from build123d import *

# Parameters (mm, degrees)
ESBO_O1_W                = 101.86
ESBO_O1_H                = 38.1
RESSALTO_EXTRUS_O1_DEPTH = 57.09
ESBO_O2_W                = 87.2
ESBO_O2_H                = 52.18
CORTE_EXTRUS_O1_DEPTH    = 57.09
ESBO_O4_W                = 3.73
ESBO_O4_H                = 12.36
CORTE_EXTRUS_O2_DEPTH    = 57.09
CORTE_EXTRUS_O3_DEPTH    = 1000
FILETE1_R                = 1
CHANFRO1_SIZE            = 2.5


with BuildPart() as part:
    # Esboço1 → Ressalto-extrusão1 (new body)
    with BuildSketch(Plane(origin=(0, 0, 0), x_dir=(1, 0, 0), z_dir=(0, 1, 0))):
        Rectangle(ESBO_O1_W, ESBO_O1_H)
    extrude(amount=RESSALTO_EXTRUS_O1_DEPTH)

    # Esboço2 → Corte-extrusão1 (cut)
    with BuildSketch(Plane.XY.offset(19.05)):
        with Locations((0, 31)):
            Rectangle(ESBO_O2_W, ESBO_O2_H)
    extrude(amount=-CORTE_EXTRUS_O1_DEPTH, mode=Mode.SUBTRACT)

    # Esboço4 → Corte-extrusão2 (cut)
    with BuildSketch(Plane.XY.offset(19.05)):
        with Locations((49.065, 50.91)):
            Rectangle(ESBO_O4_W, ESBO_O4_H)
    extrude(amount=-CORTE_EXTRUS_O2_DEPTH, mode=Mode.SUBTRACT)

    # Esboço5 → Corte-extrusão3 (cut)
    with BuildSketch(Plane(origin=(47.2, 0, 0), x_dir=(0, 0, -1), z_dir=(1, 0, 0))):
        Polygon((0, 44.73), (-12.36, 57.09), (12.36, 57.09), align=None)
    extrude(amount=-CORTE_EXTRUS_O3_DEPTH, mode=Mode.SUBTRACT)

    # Filete1
    filete1_edges = [part.edges().sort_by_distance(p)[0] for p in [
        (-47.265, 44.73, 0),
        (45.4, 44.73, 0),
    ]]
    fillet(filete1_edges, radius=FILETE1_R)

    # Chanfro1
    chanfro1_edges = [part.edges().sort_by_distance(p)[0] for p in [
        (45.4, 57.09, 19.05),
        (-47.265, 57.09, -19.05),
        (45.4, 57.09, -19.05),
        (-47.265, 57.09, 19.05),
    ]]
    chamfer(chanfro1_edges, length=CHANFRO1_SIZE)


solid = part.part
Can you work these out from the model? Positions are in its coordinate system, mm. A direction names the side the tool comes from. Coordinates: 2 decimals unless noted, no trailing zeros. Write each loop counter-clockwise with the first axis right and the second up, starting at its lowest first coordinate (ties: lowest second). Pieces come first, ordered by that corner, then holes. Notation, with made-up numbers: (31, 11) -> (65, 11) arc R12 ccw to (65, 20) -> close; hole circle Ø11 at (79.25, -36). An arc over 180 degrees is marked (long way). Write each question's results on one line, items separated by ' | '. Start each with the question number.
Item 1: If we section it at D-D, the plane z = -10: Write out the boundary of the cut face in (x, y).
Item 2: If we section it at B-B, the plane z = -15: Write out the boundary of the cut face in (x, y).
Item 3: If we section it at C-C, the plane y = 39.5: Write out the boundary of the cut face in (x, z).
Item 4: Please list where these lines run through material, in increasing order: probe 1 along X at (y, z) = (33.5, -12.5); probe 2 along X at (y, z) = (49.5, -11); probe 3 along Y at (x, z) = (36, 5.5).
Item 5: Thinking about a two-plate mould opening in X: for faces 6 (the flat face through (50.93, 22, 0)), 7 (the flat face through (-47.21, 51.18, 6.45)), 8 (the flat face through (-1, 4.91, 0)), which applies, released by +X, released by -X, zero draft, split by the parting line, or undercut?
Item 6: If we section it at A-A, the plane y = 49.5: Write out the boundary of the cut face in (x, z).
Item 7: On a 3-axis mill with a long thin cutter (end or side, diameter ignored), from which of +Z, -Z, +X, -X, +Y, -Y can I reach the whole of each face in a straight line? I mean faces 1 (the flat face through (-1, 0, 0)), 2 (the flat face through (-47, 57.09, -14)), 3 (the flat face through (-43.6, 31, 0)), 4 (the flat face through (-47.21, 51.35, -6.62)), 5 (the flat face through (47.2, 48, 5)). Say none if no direction works.
Item 8: I'm going to push flat-ended pins straight in: P1, Ø10, axis at y = 51.5, z = 9, coming from the +X side; P2, Ø11.5, axis at x = 2.5, z = -1.5, coming from the +Y side; P3, Ø4, axis at x = 48.5, z = -2, coming from the +Y side. Where does each tip first touch, or does it pass through?
Answer block:
1) outline: (-50.93, 0) -> (50.93, 0) -> (50.93, 44.73) -> (47.2, 44.73) -> (47.2, 54.73) -> (43.6, 54.73) -> (43.6, 4.91) -> (-43.6, 4.91) -> (-43.6, 54.73) -> (-50.93, 54.73) -> close
2) outline: (-50.93, 0) -> (50.93, 0) -> (50.93, 44.73) -> (47.2, 44.73) -> (47.2, 57.09) -> (43.6, 57.09) -> (43.6, 4.91) -> (-43.6, 4.91) -> (-43.6, 57.09) -> (-50.93, 57.09) -> close
3) outline: (-50.93, -19.05) -> (-43.6, -19.05) -> (-43.6, 19.05) -> (-50.93, 19.05) -> close; (43.6, -19.05) -> (50.93, -19.05) -> (50.93, 19.05) -> (43.6, 19.05) -> close
4) probe 1: -50.93 to -43.6, 43.6 to 50.93 | probe 2: -50.93 to -43.6, 43.6 to 47.2 | probe 3: 0 to 4.91
5) face 6: released by +X | face 7: zero draft | face 8: undercut
6) outline: (-50.93, -19.05) -> (-43.6, -19.05) -> (-43.6, -4.77) -> (-50.93, -4.77) -> close; (-50.93, 4.77) -> (-43.6, 4.77) -> (-43.6, 19.05) -> (-50.93, 19.05) -> close; (43.6, -19.05) -> (47.2, -19.05) -> (47.2, -4.77) -> (43.6, -4.77) -> close; (43.6, 4.77) -> (47.2, 4.77) -> (47.2, 19.05) -> (43.6, 19.05) -> close
7) face 1: +Z, -Z, +X, -X, -Y | face 2: +Z, -Z, +X, -X, +Y | face 3: +Z, -Z, +Y | face 4: +X, -X, +Y | face 5: +Z, -Z, +X, +Y
8) P1: x = 47.2 | P2: y = 4.91 | P3: y = 48.25
